Could you check a few things on this model? Use its own coordinates, in mm. Coordinates: 2 decimals unless noted, no trailing zeros. Order: outer loops, then holes, each group sorted by start corner. A loop starts at its lowest first (then second) coordinate and runs counter-clockwise, first axis right, second up. Notation, with made-up numbers: M -3,-14.5 L 5,-14.5 A29 ccw 5,7.5 Z; hole C -38.5,3 d5. An arc over 180 degrees is marked long. One line per question, with ' | ' between items. Start each with the question number.
from build123d import *

# Parameters (mm, degrees)
BOSS_EXTRUDE1_DEPTH = 0.254
SKETCH2_R           = 4.699
CUT_EXTRUDE1_DEPTH  = 1.254
SKETCH3_W           = 2.54
SKETCH3_H           = 0.635
CUT_EXTRUDE2_DEPTH  = 1.254
CUT_EXTRUDE4_DEPTH  = 1.254
SKETCH5_W           = 14.478
SKETCH5_H           = 15.24
CUT_EXTRUDE5_DEPTH  = 1.254


with BuildPart() as part:
    # Sketch1 → Boss-Extrude1 (new body)
    with BuildSketch(Plane.XY):
        with BuildLine():
            Line((67.21146711, 76.191723231), (8.696654013, 17.676910134))
            Line((8.696654013, 17.676910134), (7.228954972, 14.133571205))
            ThreePointArc((7.228954972, 14.133571205), (14.666587579, 6.075099489), (15.105587123, -4.88230096))
            Line((15.105587123, -4.88230096), (18.648926052, -6.35))
            Line((18.648926052, -6.35), (101.401368334, -6.35))
            ThreePointArc((101.401368334, -6.35), (93.866160503, 38.880636728), (67.21146711, 76.191723231))
        make_face()
        with BuildLine():
            Line((88.672924278, 6.35), (27.86051193, 6.35))
            ThreePointArc((27.86051193, 6.35), (26.399857642, 10.93517908), (24.190484974, 15.210228852))
            Line((24.190484974, 15.210228852), (67.191354125, 58.211098004))
            ThreePointArc((67.191354125, 58.211098004), (82.13289044, 34.020557137), (88.672924278, 6.35))
        make_face(mode=Mode.SUBTRACT)
    extrude(amount=BOSS_EXTRUDE1_DEPTH)

    # Sketch2 → Cut-Extrude1 (cut, through all)
    with BuildSketch(Plane.XY.offset(0.254)):
        with Locations((22.225, 0)):
            Circle(SKETCH2_R)
        with Locations((36.195, 0)):
            Circle(SKETCH2_R)
        with Locations((61.722, 0)):
            Circle(SKETCH2_R)
        with Locations((75.692, 0)):
            Circle(SKETCH2_R)
        with Locations((95.25, 0)):
            Circle(SKETCH2_R)
        with Locations((15.715448212, 15.715448212)):
            Circle(SKETCH2_R)
        with Locations((25.593729945, 25.593729945)):
            Circle(SKETCH2_R)
        with Locations((43.644044748, 43.644044748)):
            Circle(SKETCH2_R)
        with Locations((53.522326482, 53.522326482)):
            Circle(SKETCH2_R)
        with Locations((92.004434954, 24.652514046)):
            Circle(SKETCH2_R)
        with Locations((82.48891971, 47.625)):
            Circle(SKETCH2_R)
        with Locations((67.351920908, 67.351920908)):
            Circle(SKETCH2_R)
    extrude(amount=-CUT_EXTRUDE1_DEPTH, mode=Mode.SUBTRACT)

    # Sketch3 → Cut-Extrude2 (cut, through all)
    with BuildSketch(Plane.XY.offset(0.254)):
        Polygon((15.266435406, 24.246691527), (17.06248663, 26.042742751), (17.511499436, 25.593729945), (15.715448212, 23.797678721), align=None)
        Polygon((44.991083167, 53.971339288), (43.195031942, 52.175288063), (43.644044748, 51.726275257), (45.440095973, 53.522326482), align=None)
        with Locations((29.21, -6.0325)):
            Rectangle(SKETCH3_W, SKETCH3_H)
        with Locations((68.707, -6.0325)):
            Rectangle(SKETCH3_W, SKETCH3_H)
        Polygon((29.230733674, 38.210989795), (31.026784898, 40.007041019), (31.475797704, 39.558028213), (29.67974648, 37.761976989), align=None)
        Polygon((56.845021246, 65.825277367), (55.048970022, 64.029226143), (55.497982828, 63.580213337), (57.294034052, 65.376264561), align=None)
        with Locations((48.9585, -6.0325)):
            Rectangle(SKETCH3_W, SKETCH3_H)
        with Locations((85.471, -6.0325)):
            Rectangle(SKETCH3_W, SKETCH3_H)
        Polygon((99.935462164, 14.437711971), (100.266998693, 11.919442024), (101.526133667, 12.085210288), (101.194597138, 14.603480236), align=None)
        Polygon((93.765504959, 37.464305742), (94.938831965, 37.950313702), (93.966816047, 40.296967714), (92.793489041, 39.810959755), align=None)
        Polygon((79.327792988, 62.471156422), (80.874047017, 60.456038938), (81.88160576, 61.229165953), (80.33535173, 63.244283437), align=None)
        Polygon((13.593916116, 7.005422516), (14.565932035, 4.658768503), (15.739259041, 5.144776462), (14.767243123, 7.491430475), align=None)
    extrude(amount=-CUT_EXTRUDE2_DEPTH, mode=Mode.SUBTRACT)

    # Sketch6 → Cut-Extrude4 (cut, through all)
    with BuildSketch(Plane.XY.offset(0.254)):
        with BuildLine():
            Line((22.27103518, 28.91642471), (40.321349984, 46.966739513))
            ThreePointArc((40.321349984, 46.966739513), (46.966739513, 46.966739513), (46.966739513, 40.321349984))
            Line((46.966739513, 40.321349984), (28.91642471, 22.27103518))
            ThreePointArc((28.91642471, 22.27103518), (22.27103518, 22.27103518), (22.27103518, 28.91642471))
        make_face()
        with BuildLine():
            Line((50.199631717, 56.845021246), (64.029226143, 70.674615673))
            ThreePointArc((64.029226143, 70.674615673), (70.674615673, 70.674615673), (70.674615673, 64.029226143))
            Line((70.674615673, 64.029226143), (56.845021246, 50.199631717))
            ThreePointArc((56.845021246, 50.199631717), (50.199631717, 50.199631717), (50.199631717, 56.845021246))
        make_face()
        with BuildLine():
            Line((61.722, -4.699), (36.195, -4.699))
            ThreePointArc((36.195, -4.699), (31.496, 0), (36.195, 4.699))
            Line((36.195, 4.699), (61.722, 4.699))
            ThreePointArc((61.722, 4.699), (66.421, 0), (61.722, -4.699))
        make_face()
        with BuildLine():
            ThreePointArc((26.924, 0), (24.874532533, 10.303368733), (19.038142977, 19.038142977))
            ThreePointArc((19.038142977, 19.038142977), (12.392753447, 19.038142977), (12.392753447, 12.392753447))
            ThreePointArc((12.392753447, 12.392753447), (16.191912687, 6.706909836), (17.526, 0))
            ThreePointArc((17.526, 0), (22.225, -4.699), (26.924, 0))
        make_face()
        with BuildLine():
            ThreePointArc((96.543320412, 25.868704739), (92.340835395, 38.248826381), (86.558373083, 49.9745))
            ThreePointArc((86.558373083, 49.9745), (80.13941971, 51.694453372), (78.419466338, 45.2755))
            ThreePointArc((78.419466338, 45.2755), (83.658215548, 34.652367484), (87.465549496, 23.436323353))
            ThreePointArc((87.465549496, 23.436323353), (93.220625647, 20.113628588), (96.543320412, 25.868704739))
        make_face()
    extrude(amount=-CUT_EXTRUDE4_DEPTH, mode=Mode.SUBTRACT)

    # Sketch5 → Cut-Extrude5 (cut, through all)
    with BuildSketch(Plane.XY.offset(0.254)):
        with Locations((77.089, 0)):
            Rectangle(SKETCH5_W, SKETCH5_H)
    extrude(amount=-CUT_EXTRUDE5_DEPTH, mode=Mode.SUBTRACT)


solid = part.part
(1) Imagine slicing it at C-C, the plane x = 75. Write out the boundary of the cut face in (y, z), plus the area to 3 significant figures.
(2) Imagine slicing it at A-A, the plane y = 33.5. Write out the boundary of the cut face in (x, z).
(3) Imagine slicing it at B-B, the plane z = 0.1. Count the separate pieces of the cut face and the enclosed holes in it, plus the area to 3 significant figures.
(4) If I drill on line 1 along Y through (x, z) = (37, 0.15); line 2 along X through (y, z) = (28, 0.1); line 3 along X through (y, z) = (3, 0.05), over which ranges is the centre line in solid material (lowest first)? Write a range as from..to.
Answers:
1) outline: M 47.73,0 L 68.54,0 L 68.54,0.25 L 47.73,0.25 Z | area: 5.29 mm²
2) outline: M 24.52,0 L 26.85,0 L 26.85,0.25 L 24.52,0.25 Z; M 40.15,0 L 42.48,0 L 42.48,0.25 L 40.15,0.25 Z; M 82.35,0 L 84.13,0 L 84.13,0.25 L 82.35,0.25 Z; M 94.17,0 L 95.92,0 L 95.92,0.25 L 94.17,0.25 Z
3) separate pieces: 1 | enclosed holes: 6 | area: 1,350 mm²
4) line 1: -6.35..-4.7, 4.7..6.35, 28.02..30.35, 43.65..45.98 | line 2: 19.02..21.56, 34.65..36.98, 84.38..86.11, 95.95..97.67 | line 3: 15.59..17.27, 26.76..32.58, 65.34..69.85, 84.33..91.63, 98.87..101.56
